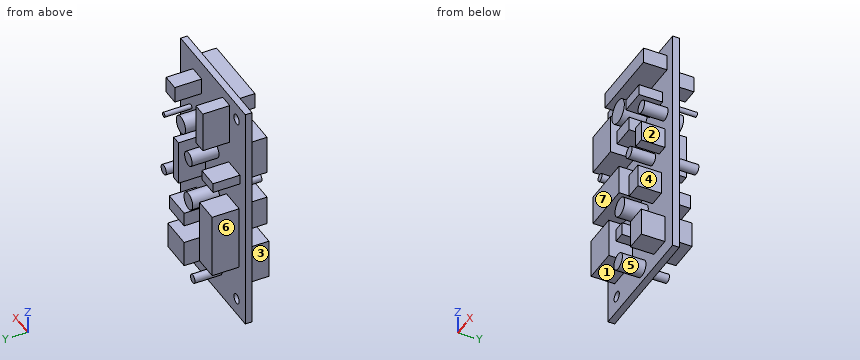
Autodesk Inventor part; units mm, degrees
ref_plane "YZ Plane" through (0, 0, 0) normal (1, 0, 0) x (0, 1, 0)
ref_plane "XZ Plane" through (0, 0, 0) normal (0, 1, 0) x (-1, 0, 0)
ref_plane "XY Plane" through (0, 0, 0) normal (0, 0, 1) x (1, 0, 0)
sketch "Sketch1" plane through (0, 0, 0) normal (0, 1, 0) x (-1, 0, 0)
  line L0 (0, 0) -> (37, 0)
  line L1 (37, 0) -> (37, -70)
  line L2 (37, -70) -> (0, -70)
  line L3 (0, -70) -> (0, 0)
  dimension "d0" = 37
  dimension "d1" = 70
extrude "Extrusion1" add sketch "Sketch1" along normal blind 2
sketch "Sketch2" plane through (0, 2, 0) normal (0, 1, 0) x (1, 0, 0)
  circle A0 centre (-32, 5) radius 1.5
  circle A1 centre (-32, 65) radius 1.5
  line L0 (-37, 70) -> (-37, 0)
  line L1 (-37, 0) -> (0, 0)
  line L2 (0, 70) -> (-37, 70)
  dimension "d4" = 3
  dimension "d5" = 3
  dimension "d6" = 5
  dimension "d11" = 60
  dimension "d12" = 5
extrude "Extrusion2" cut sketch "Sketch2" against normal through all
sketch "Sketch3" plane through (0, 2, 0) normal (0, 1, 0) x (1, 0, 0)
  line L0 (-8.0701, 61.2061) -> (-17.4041, 61.2061)
  line L1 (-17.4041, 61.2061) -> (-17.4041, 53.4277)
  line L2 (-17.4041, 53.4277) -> (-8.0701, 53.4277)
  line L3 (-8.0701, 53.4277) -> (-8.0701, 61.2061)
  line L4 (-26.252, 53.4277) -> (-33.447, 53.4277)
  line L5 (-33.447, 53.4277) -> (-33.447, 33.8845)
  line L6 (-33.447, 33.8845) -> (-26.252, 33.8845)
  line L7 (-26.252, 33.8845) -> (-26.252, 53.4277)
  line L8 (-14.1955, 35.8291) -> (-11.4731, 35.8291)
  line L9 (-11.4731, 35.8291) -> (-11.4731, 22.3142)
  line L10 (-11.4731, 22.3142) -> (-14.1955, 22.3142)
  line L11 (-14.1955, 22.3142) -> (-14.1955, 35.8291)
  line L12 (-8.9451, 47.8856) -> (-17.4041, 47.8856)
  line L13 (-17.4041, 47.8856) -> (-17.4041, 43.6561)
  line L14 (-17.4041, 43.6561) -> (-8.9451, 43.6561)
  line L15 (-8.9451, 43.6561) -> (-8.9451, 47.8856)
  line L16 (-7.0978, 10.1605) -> (-12.0565, 10.1605)
  line L17 (-12.0565, 10.1605) -> (-12.0565, 5.299)
  line L18 (-12.0565, 5.299) -> (-7.0978, 5.299)
  line L19 (-7.0978, 5.299) -> (-7.0978, 10.1605)
  line L20 (-24.113, 3.0627) -> (-28.0994, 3.0627)
  line L21 (-28.0994, 3.0627) -> (-28.0994, 15.3137)
  line L22 (-28.0994, 15.3137) -> (-24.113, 15.3137)
  line L23 (-24.113, 15.3137) -> (-24.113, 3.0627)
  line L24 (-27.516, 22.3142) -> (-33.9332, 22.3142)
  line L25 (-33.9332, 22.3142) -> (-33.9332, 25.2311)
  line L26 (-33.9332, 25.2311) -> (-27.516, 25.2311)
  line L27 (-27.516, 25.2311) -> (-27.516, 22.3142)
  circle A0 centre (-19.8349, 37.871) radius 2.5092
  circle A1 centre (-19.8349, 23.7727) radius 2.1324
  circle A2 centre (-5.7366, 37.1904) radius 1.481
  circle A3 centre (-5.7366, 18.8139) radius 0.7011
  circle A4 centre (-15.5567, 15.3137) radius 2.6288
  circle A5 centre (-22.3441, 62.1784) radius 1.2864
  point P0 (0, 0)
extrude "Extrusion3" add sketch "Sketch3" along normal blind 8
sketch "Sketch4" plane through (0, 0, 0) normal (0, -1, 0) x (1, 0, 0)
  line L0 (-18.8626, -58.0947) -> (-15.5567, -58.0947)
  line L1 (-15.5567, -58.0947) -> (-15.5567, -54.2055)
  line L2 (-15.5567, -54.2055) -> (-18.8626, -54.2055)
  line L3 (-18.8626, -54.2055) -> (-18.8626, -58.0947)
  line L4 (-18.3764, -25.9117) -> (-11.4731, -25.9117)
  line L5 (-11.4731, -25.9117) -> (-11.4731, -21.7308)
  line L6 (-11.4731, -21.7308) -> (-18.3764, -21.7308)
  line L7 (-18.3764, -21.7308) -> (-18.3764, -25.9117)
  line L8 (-6.4172, -48.1773) -> (-11.4731, -48.1773)
  line L9 (-11.4731, -48.1773) -> (-11.4731, -41.274)
  line L10 (-11.4731, -41.274) -> (-6.4172, -41.274)
  line L11 (-6.4172, -41.274) -> (-6.4172, -48.1773)
  line L12 (-32.0858, -34.1762) -> (-17.2097, -34.1762)
  line L13 (-17.2097, -34.1762) -> (-17.2097, -43.0241)
  line L14 (-17.2097, -43.0241) -> (-32.0858, -43.0241)
  line L15 (-32.0858, -43.0241) -> (-32.0858, -34.1762)
  line L16 (-33.1553, -59.9421) -> (-23.0434, -59.9421)
  line L17 (-23.0434, -59.9421) -> (-23.0434, -48.1773)
  line L18 (-23.0434, -48.1773) -> (-33.1553, -48.1773)
  line L19 (-33.1553, -48.1773) -> (-33.1553, -59.9421)
  line L20 (-32.0858, -25.9117) -> (-22.0711, -25.9117)
  line L21 (-22.0711, -25.9117) -> (-22.0711, -14.1469)
  line L22 (-22.0711, -14.1469) -> (-32.0858, -14.1469)
  line L23 (-32.0858, -14.1469) -> (-32.0858, -25.9117)
  line L24 (-25.1825, -4.3267) -> (-3.2086, -4.3267)
  line L25 (-3.2086, -4.3267) -> (-3.2086, -9.091)
  line L26 (-3.2086, -9.091) -> (-25.1825, -9.091)
  line L27 (-25.1825, -9.091) -> (-25.1825, -4.3267)
  circle A0 centre (-5.7366, -18.8139) radius 0.7011
  line L28 (-13.2232, -14.8275) -> (-5.7366, -14.8275)
  line L29 (-5.7366, -14.8275) -> (-5.7366, -18.1128)
  line L30 (-5.7366, -18.1128) -> (-13.2232, -18.1128)
  line L31 (-13.2232, -18.1128) -> (-13.2232, -14.8275)
  line L32 (-7.6811, -34.1762) -> (-4.4726, -34.1762)
  line L33 (-4.4726, -34.1762) -> (-4.4726, -27.9535)
  line L34 (-4.4726, -27.9535) -> (-7.6811, -27.9535)
  line L35 (-7.6811, -27.9535) -> (-7.6811, -34.1762)
  line L36 (-10.6953, -65.6787) -> (-4.4726, -65.6787)
  line L37 (-4.4726, -65.6787) -> (-4.4726, -57.3169)
  line L38 (-4.4726, -57.3169) -> (-10.6953, -57.3169)
  line L39 (-10.6953, -57.3169) -> (-10.6953, -65.6787)
  circle A1 centre (-17.6958, -65.6787) radius 2.4366
  circle A2 centre (-16.7235, -48.1773) radius 2.7842
  circle A3 centre (-11.4731, -33.4956) radius 1.7008
  circle A4 centre (-28.0994, -30.3843) radius 1.1308
  circle A5 centre (-17.6958, -15.5081) radius 3.5421
  circle A6 centre (-4.4726, -23.092) radius 1.8576
  point P0 (0, 0)
extrude "Extrusion4" add sketch "Sketch4" along normal blind 7 contours L3 L2 L1 L0 | L7 L6 L5 L4 | L8 L9 L10 L11 | L12 L13 L14 L15 | L19 L18 L17 L16 | L23 L22 L21 L20 | L24 L25 L26 L27 | L30 L31 L28 L29 | L35 L34 L33 L32 | L39 L38 L37 L36 | A1 | A2 | A3 | A4 | A5 | A6
properties part number "printplaat"
Geometry: final body of the model. Coordinates: model frame, mm. Face numbers are marked on the shaded views. A direction names the side the tool comes from. Coordinates: 2 decimals unless noted, no trailing zeros. Write each loop counter-clockwise with the first axis right and the second up, starting at its lowest first coordinate (ties: lowest second). Pieces come first, ordered by that corner, then holes. Notation, with made-up numbers: M 66.25,46.25 L 97.25,46.25 A13 ccw 97.25,71.25 Z; hole C 70,50 d1. An arc over 180 degrees is marked long. Answer as CSV lines item,"result". Start each with the question number.
Q1. Line query: line 1 (Z direction, x = -6.5, y = -6); line 2 (Z direction, x = -32, y = 1.4); line 3 (Z direction, x = -8.5, y = -1.5). Output: solid intervals per line, ascending. Write a range as from..to.
Q2. Cut plane B-B on y = 5.75. Count the separate pieces of the cut face and the enclosed holes in it, then the cut area to 3 significant figures.
Q3. Cut plane A-A on z = -65. Return the cut outline in (x, y), then the cut area to 3 significant figures.
Q4. Reachability of the marked faces 1, 2, 3 and 4 from +Z, -Z, +X, -X, +Y, -Y: full face, straight path, thin tool, end or side. Return the list, or none.
Q5. Cut plane C-C on z = -8. Return the cut outline in (x, y).
Q6. Pin query (flat end, axial travel): P1, Ø3.5, axis at y = 6.5, z = -45, coming from the +X side; P2, Ø4, axis at x = -8.5, y = -2.5, coming from the -Z side; P3, Ø6.5, axis at y = 7, z = -12, coming from the +X side. Return the tip coordinate at first contact, or that it passes through.
Q7. Mould query, pull axis X, two halves, no side actions, for the marked faces 5, 6 and 7. Classes: released by +X, released by -X, zero draft, split by the parting line, or undercut.
Findings below:
1,line 1,"z = -65.68..-57.32, -48.18..-41.27, -34.18..-27.95, -18.11..-14.83, -9.09..-4.33"
1,line 2,"z = -70..-66.5, -63.5..-6.5, -3.5..0"
1,line 3,"z = -65.68..-57.32, -48.18..-41.27, -18.11..-14.83, -9.09..-4.33"
2,separate pieces,"13"
2,enclosed holes,"0"
2,area,"447 mm2"
3,outline,"M -37,0 L -33.5,0 L -33.5,2 L -37,2 Z; M -30.5,0 L -20.04,0 L -20.04,-7 L -15.36,-7 L -15.36,0 L -10.7,0 L -10.7,-7 L -4.47,-7 L -4.47,0 L 0,0 L 0,2 L -30.5,2 Z"
3,area,"144 mm2"
4,face 1,"-Z, -X, -Y"
4,face 2,"-Z, +X, -Y"
4,face 3,"+Z, -Z, -X, -Y"
4,face 4,"+X, -Y"
5,outline,"M -37,0 L -25.18,0 L -25.18,-7 L -3.21,-7 L -3.21,0 L 0,0 L 0,2 L -7.1,2 L -7.1,10 L -12.06,10 L -12.06,2 L -24.11,2 L -24.11,10 L -28.1,10 L -28.1,2 L -37,2 Z"
6,P1,"stops at x = -8.95"
6,P2,"stops at z = -65.68"
6,P3,"stops at x = -7.1"
7,face 5,"undercut"
7,face 6,"released by -X"
7,face 7,"zero draft"
